Verification items for the finished model (mm, model axes). A direction names the side the tool comes from. Round coordinates to 2 decimals unless told otherwise and drop trailing zeros. Loops run counter-clockwise (first coordinate to the right, second up) from the corner with the lowest first, then second, coordinate; pieces in that order, holes last. Notation, with made-up numbers: (-34.75, 71) -> (1.25, 71) arc R19 ccw to (1.25, 105) -> close; hole circle Ø10 at (12.5, 49). An arc over 180 degrees is marked (long way). Use a Markdown table: item, result. Add a question column.
```python
from build123d import *

# Parameters (mm, degrees)
CROQUIS1_W               = 180
CROQUIS1_H               = 64.6
SALIENTE_EXTRUIR1_DEPTH  = 5
CROQUIS2_W               = 10
CROQUIS2_H               = 5
SALIENTE_EXTRUIR2_DEPTH  = 5
REDONDEO1_R              = 0.5
REDONDEO1_OF_SIMETR_A1_R = 0.5
REDONDEO2_R              = 10
CROQUIS3_W               = 130
CROQUIS3_H               = 34.6
CORTAR_EXTRUIR1_DEPTH    = 5
REDONDEO3_R              = 3


with BuildPart() as part:
    # Croquis1 → Saliente-Extruir1 (new body)
    with BuildSketch(Plane.XY):
        Rectangle(CROQUIS1_W, CROQUIS1_H)
    extrude(amount=SALIENTE_EXTRUIR1_DEPTH)

    # Croquis2 → Saliente-Extruir2 (add)
    with BuildSketch(Plane(origin=(0, 32.3, 0), x_dir=(1, 0, 0), z_dir=(0, 1, 0))):
        with Locations((-60, -2.5)):
            Rectangle(CROQUIS2_W, CROQUIS2_H)
        with Locations((-10, -2.5)):
            Rectangle(CROQUIS2_W, CROQUIS2_H)
        with Locations((40, -2.5)):
            Rectangle(CROQUIS2_W, CROQUIS2_H)
    saliente_extruir2 = extrude(amount=SALIENTE_EXTRUIR2_DEPTH)

    # Redondeo1
    redondeo1_edges = [part.edges().sort_by_distance(p)[0] for p in [
        (-65, 34.8, 0),
        (-65, 34.8, 5),
        (-55, 34.8, 5),
        (-55, 34.8, 0),
        (-65, 37.3, 2.5),
        (-60, 37.3, 5),
        (-55, 37.3, 2.5),
        (-60, 37.3, 0),
        (-15, 34.8, 0),
        (-15, 34.8, 5),
        (-5, 34.8, 5),
        (-5, 34.8, 0),
        (-15, 37.3, 2.5),
        (-10, 37.3, 5),
        (-5, 37.3, 2.5),
        (-10, 37.3, 0),
        (35, 34.8, 0),
        (35, 34.8, 5),
        (45, 34.8, 5),
        (45, 34.8, 0),
        (35, 37.3, 2.5),
        (40, 37.3, 5),
        (45, 37.3, 2.5),
        (40, 37.3, 0),
    ]]
    fillet(redondeo1_edges, radius=REDONDEO1_R)

    # Simetría1: Saliente-Extruir2 across plane
    add(saliente_extruir2.mirror(Plane.ZX))

    # Redondeo1 of Simetría1
    redondeo1_of_simetr_a1_edges = [part.edges().sort_by_distance(p)[0] for p in [
        (-65, -34.8, 0),
        (-65, -34.8, 5),
        (-55, -34.8, 5),
        (-55, -34.8, 0),
        (-65, -37.3, 2.5),
        (-60, -37.3, 5),
        (-55, -37.3, 2.5),
        (-60, -37.3, 0),
        (-15, -34.8, 0),
        (-15, -34.8, 5),
        (-5, -34.8, 5),
        (-5, -34.8, 0),
        (-15, -37.3, 2.5),
        (-10, -37.3, 5),
        (-5, -37.3, 2.5),
        (-10, -37.3, 0),
        (35, -34.8, 0),
        (35, -34.8, 5),
        (45, -34.8, 5),
        (45, -34.8, 0),
        (35, -37.3, 2.5),
        (40, -37.3, 5),
        (45, -37.3, 2.5),
        (40, -37.3, 0),
    ]]
    fillet(redondeo1_of_simetr_a1_edges, radius=REDONDEO1_OF_SIMETR_A1_R)

    # Redondeo2
    redondeo2_edges = [part.edges().sort_by_distance(p)[0] for p in [
        (90, 32.3, 2.5),
        (90, -32.3, 2.5),
    ]]
    fillet(redondeo2_edges, radius=REDONDEO2_R)

    # Croquis3 → Cortar-Extruir1 (cut)
    with BuildSketch(Plane(origin=(0, 0, 0), x_dir=(-1, 0, 0), z_dir=(0, 0, -1))):
        with Locations((10, 0)):
            Rectangle(CROQUIS3_W, CROQUIS3_H)
    extrude(amount=-CORTAR_EXTRUIR1_DEPTH, mode=Mode.SUBTRACT)

    # Redondeo3
    redondeo3_edges = [part.edges().sort_by_distance(p)[0] for p in [
        (55, -17.3, 2.5),
        (55, 17.3, 2.5),
        (-75, 17.3, 2.5),
        (-75, -17.3, 2.5),
    ]]
    fillet(redondeo3_edges, radius=REDONDEO3_R)


solid = part.part
```
1) Sectioned sample at D-D on x = 59.5. Enter the section's corners in (y, z).
2) Go/stop test with flat-tipped pins: pin 1 (2 mm diameter, centred on x = -17, z = 3.5, fed in from +Y); pin 2 (2.5 mm diameter, centred on x = -34, z = 3.5, fed in from -Y); pin 3 (1.2 mm diameter, centred on y = 33.5, z = 2.5, fed in from +X); pin 4 (10 mm diameter, centred on x = -48.5, y = 12, fed in from -Z). Record where each tip stops, or that it passes through.
3) Release check for a two-part mould opening along Y. For faces 6 (the face through (-75, 0, 2)), 7 (the face through (90, 0, 2)), 8 (the face through (-35, -32.3, 2)) record: released by +Y, released by -Y, zero draft, split by the parting line, or undercut.
4) Thickness scan on line 1 (X direction, y = 4, z = 4.25); line 2 (Y direction, x = -25, z = 0.45); line 3 (X direction, y = -23, z = 2.85). Record the ranges inside material, lowest first.
5) Sectioned sample at C-C on x = -40. Enter the section's corners in (y, z), then the cut area to 3 significant figures.
6) Sectioned sample at A-A on x = -10.5. Enter the section's corners in (y, z), then the cut area to 3 significant figures.
7) Access from +Z, -Z, +X, -X, +Y, -Y to the whole of each face (thin tool, end or side, straight path). Record for faces 1 (the face through (-65, 35, 3)), 2 (the face through (-74.1, 16.44, 2.54)), 3 (the face through (-55, -35, 3)), 4 (the face through (45, -35, 3)), 5 (the face through (-5, 35, 3)).
8) Sectioned sample at B-B on y = -10. Enter the section's corners in (x, z).
Geometry results:
| question | item | result |
|---|---|---|
| 1 | outline | (-32.3, 0) -> (32.3, 0) -> (32.3, 5) -> (-32.3, 5) -> close |
| 2 | pin 1 | y = 32.3 |
| 2 | pin 2 | y = -32.3 |
| 2 | pin 3 | x = 45 |
| 2 | pin 4 | through |
| 3 | face 6 | undercut |
| 3 | face 7 | zero draft |
| 3 | face 8 | released by -Y |
| 4 | line 1 | -90 to -75, 55 to 90 |
| 4 | line 2 | -32.3 to -17.3, 17.3 to 32.3 |
| 4 | line 3 | -90 to 89.98 |
| 5 | outline | (-32.3, 0) -> (-17.3, 0) -> (-17.3, 5) -> (-32.3, 5) -> close; (17.3, 0) -> (32.3, 0) -> (32.3, 5) -> (17.3, 5) -> close |
| 5 | area | 150 mm^2 |
| 6 | outline | (-37.3, 0.5) arc R0.5 ccw to (-36.8, 0) -> (-17.3, 0) -> (-17.3, 5) -> (-36.8, 5) arc R0.5 ccw to (-37.3, 4.5) -> close; (17.3, 0) -> (36.8, 0) arc R0.5 ccw to (37.3, 0.5) -> (37.3, 4.5) arc R0.5 ccw to (36.8, 5) -> (17.3, 5) -> close |
| 6 | area | 200 mm^2 |
| 7 | face 1 | +Z, -Z, -X, +Y |
| 7 | face 2 | +Z, -Z |
| 7 | face 3 | +Z, -Z, -Y |
| 7 | face 4 | +Z, -Z, +X, -Y |
| 7 | face 5 | +Z, -Z, +Y |
| 8 | outline | (-90, 0) -> (-75, 0) -> (-75, 5) -> (-90, 5) -> close; (55, 0) -> (90, 0) -> (90, 5) -> (55, 5) -> close |
